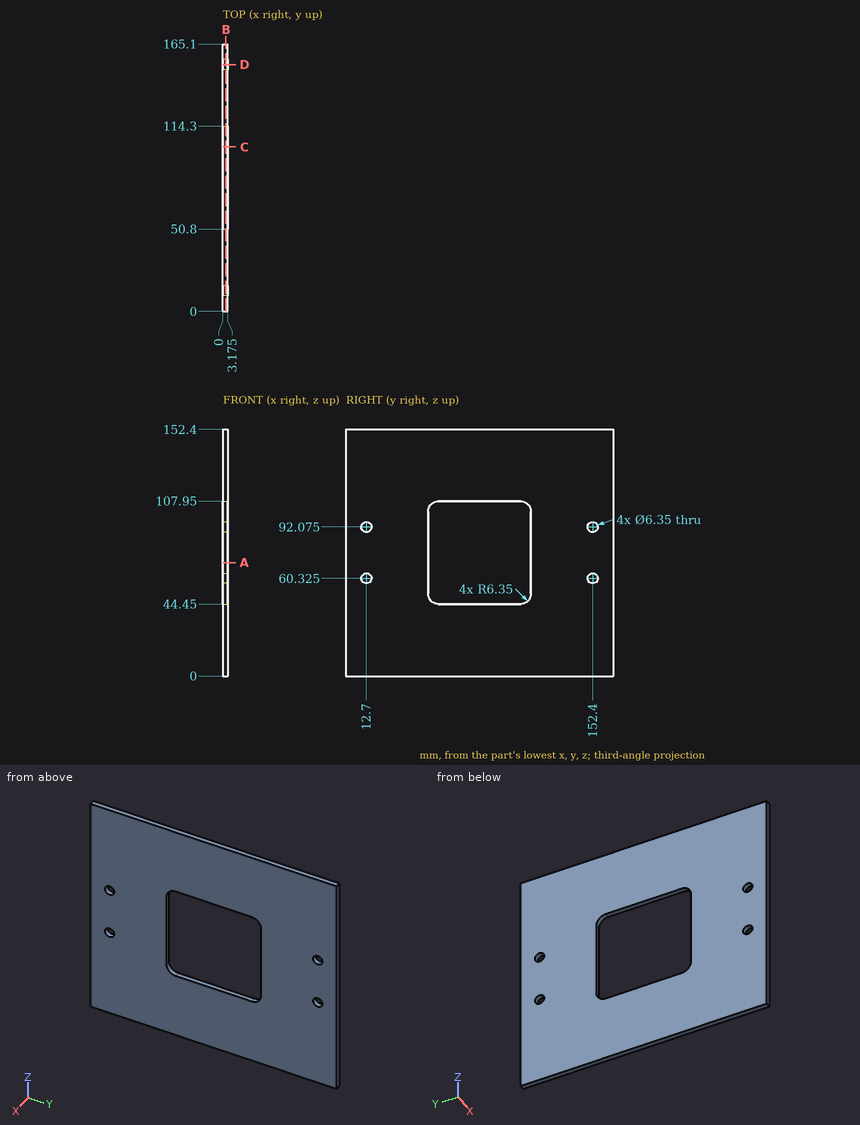
Verification items for this drawing (mm, ordinates from the low corner). Round coordinates to 2 decimals unless told otherwise and drop trailing zeros. Loops run counter-clockwise (first coordinate to the right, second up) from the corner with the lowest first, then second, coordinate; pieces in that order, holes last. Notation, with made-up numbers: M -25.75,-26 L 14.25,-26 A36 cw 14.25,12 Z; hole C 23.5,-4 d4. An arc over 180 degrees is marked long. Answer as a JSON object with one key per item and string values.
1. Scan lines: line 1 (Y direction, x = 0.1, z = 56.5); line 2 (Z direction, x = 2.8, y = 59); line 3 (Y direction, x = 1.2, z = 106). Record each from-to range of solid material in increasing order.
Reply:
{"line 1": "y = 0 to 50.8, 114.3 to 165.1", "line 2": "z = 0 to 44.45, 107.95 to 152.4", "line 3": "y = 0 to 52.57, 112.53 to 165.1"}
2. Section check A-A (z = 70). Record the boundary of the cut face in (x, y) (3 decimals).
Reply:
{"outline": "M 0,0 L 3.175,0 L 3.175,50.8 L 0,50.8 Z; M 0,114.3 L 3.175,114.3 L 3.175,165.1 L 0,165.1 Z"}
3. Section check B-B (x = 1.85). Record the boundary of the cut face in (y, z) (3 decimals), plus the area to 3 significant figures.
Reply:
{"outline": "M 0,0 L 165.1,0 L 165.1,152.4 L 0,152.4 Z; hole C 12.7,60.325 d6.35; hole C 12.7,92.075 d6.35; hole M 50.8,50.8 A6.35 ccw 57.15,44.45 L 107.95,44.45 A6.35 ccw 114.3,50.8 L 114.3,101.6 A6.35 ccw 107.95,107.95 L 57.15,107.95 A6.35 ccw 50.8,101.6 Z; hole C 152.4,60.325 d6.35; hole C 152.4,92.075 d6.35", "area": "21,000 mm²"}
4. Section check D-D (y = 152.4). Record the boundary of the cut face in (x, z) (3 decimals).
Reply:
{"outline": "M 0,0 L 3.175,0 L 3.175,57.15 L 0,57.15 Z; M 0,63.5 L 3.175,63.5 L 3.175,88.9 L 0,88.9 Z; M 0,95.25 L 3.175,95.25 L 3.175,152.4 L 0,152.4 Z"}
5. Section check C-C (y = 101.5). Record the boundary of the cut face in (x, z) (3 decimals), plus the area to 3 significant figures.
Reply:
{"outline": "M 0,0 L 3.175,0 L 3.175,44.45 L 0,44.45 Z; M 0,107.95 L 3.175,107.95 L 3.175,152.4 L 0,152.4 Z", "area": "282 mm²"}
